Verification items for this drawing (mm, ordinates from the low corner). A direction names the side the tool comes from. Coordinates: 2 decimals unless noted, no trailing zeros. Order: outer loops, then holes, each group sorted by start corner. A loop starts at its lowest first (then second) coordinate and runs counter-clockwise, first axis right, second up. Notation, with made-up numbers: (23.5, 6) -> (38.5, 6) arc R21 cw to (38.5, 30) -> close; hole circle Ø7 at (74.25, 77). An arc over 180 degrees is marked (long way). Write item = value, one per line. Start each with the question number.
1. Release check for a two-part mould opening along X. For the marked faces 1, 2 and 3 record: +X half, -X half, draft (parallel to the pull), parting line (faces both ways), or undercut.
2. Cross-section at B-B on x = 80. Record the cut outline in (y, z).
3. Thickness scan on line 1 along Y through (x, z) = (80, 8); line 2 along Y through (x, z) = (248, 19); line 3 along Z through (x, y) = (110.5, 22). Record the ranges inside material, lowest first. Write a range as from..to.
4. Cross-section at C-C on x = 248. Record the cut outline in (y, z).
5. Go/stop test with flat-tipped pins: P1, Ø4, axis at x = 142.5, z = 92.5, coming from the -Y side; P2, Ø4, axis at y = 88.5, z = 18, coming from the +X side; P3, Ø3, axis at y = 219.5, z = 150, coming from the +X side. Record where each tip stops, or that it passes through.
6. Cross-section at D-D on z = 83.5. Record the cut outline in (x, y).
7. Set-up check for the marked faces 4, 5, 6, 7 and 8: record each of +Z, -Z, +X, -X, +Y, -Y from which the full face is reachable in a straight line by a thin tool's end or side.
8. Cross-section at A-A on y = 240. Record the cut outline in (x, z).
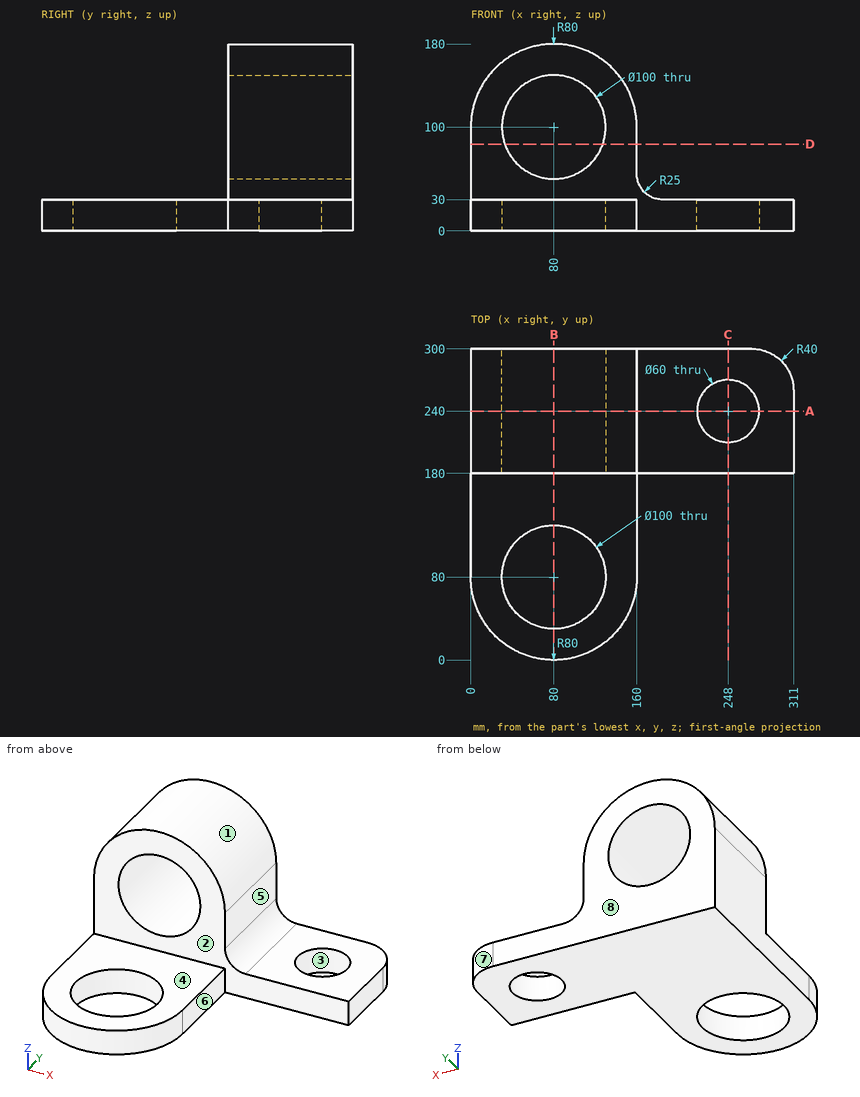
Worked out:
q1.face_1 = parting line
q1.face_2 = draft
q1.face_3 = undercut
q2.outline = (0, 0) -> (30, 0) -> (30, 30) -> (0, 30) -> close; (130, 0) -> (300, 0) -> (300, 50) -> (180, 50) -> (180, 30) -> (130, 30) -> close; (180, 150) -> (300, 150) -> (300, 180) -> (180, 180) -> close
q3.line_1 = 0..30, 130..300
q3.line_2 = 180..210, 270..300
q3.line_3 = 0..30
q4.outline = (180, 0) -> (210, 0) -> (210, 30) -> (180, 30) -> close; (270, 0) -> (300, 0) -> (300, 30) -> (270, 30) -> close
q5.P1 = 180
q5.P2 = 160
q5.P3 = 143.62
q6.outline = (0, 180) -> (32.8, 180) -> (32.8, 300) -> (0, 300) -> close; (127.2, 180) -> (160, 180) -> (160, 300) -> (127.2, 300) -> close
q7.face_4 = +Z, +X, -X, -Y
q7.face_5 = +Z, +X, +Y, -Y
q7.face_6 = +Z, -Z, +X, -Y
q7.face_7 = +Z, -Z, +X, +Y
q7.face_8 = +Z, -Z, +X, -X, +Y
q8.outline = (0, 0) -> (218, 0) -> (218, 30) -> (185, 30) arc R25 cw to (160, 55) -> (160, 100) arc R80 ccw to (0, 100) -> close; (278, 0) -> (311, 0) -> (311, 30) -> (278, 30) -> close; hole circle Ø100 at (80, 100)
